Could you check a few things on this model? Use its own coordinates, in mm. Face numbers are marked on the shaded views. Round coordinates to 2 decimals unless told otherwise and drop trailing zeros. Loops run counter-clockwise (first coordinate to the right, second up) from the corner with the lowest first, then second, coordinate; pieces in that order, holes last. Notation, with made-up numbers: M -22.75,17.5 L 9.25,17.5 A19 ccw 9.25,38.5 Z; hole C 85.5,-27.75 d11. An arc over 180 degrees is marked long. One line per item, written item: value. Start each with the question number.
Q1. Imagine slicing it at B-B (z = 4.5). Please give me the cut outline in (x, y).
Q2. Imagine slicing it at D-D (z = 9.25). Give the number of separate pieces and of enclosed holes in the cut face, then the cut area to 3 significant figures.
Q3. Imagine slicing it at A-A (y = 51). Please give me the cut outline in (x, z), then the cut area to 3 significant figures.
Q4. Imagine slicing it at C-C (x = 21). Please give me the cut outline in (y, z), then the cut area to 3 significant figures.
Q5. I'm going to push flat-ended pins straight in: pin 1 Ø2 at (x, y) = (20.5, 37) entering from +Z; pin 2 Ø5 at (x, z) = (5.5, 6) entering from +Y; pin 3 Ø1 at (x, z) = (6.5, 3) entering from -Y. Where does each tip first touch, or does it pass through?
Q6. Please list where these lines run through material, in increasing order: line 1 along X through (y, z) = (39, 8.5); line 2 along X through (y, z) = (20, 8.25); line 3 along Y through (x, z) = (22, 8.25).
Q7. Thinking about a two-plate mould opening in X: for the marked faces 1, 2, 3 and 4, which applies, released by +X, released by -X, zero draft, split by the parting line, or undercut?
from build123d import *

# Parameters (mm, degrees)
EXTRUDE1_DEPTH = 10.16
CHAMFER1_SIZE  = 2.54
FILLET1_R      = 2.54
SKETCH2_R      = 2.50622178
SKETCH2_W      = 20.082955398
SKETCH2_H      = 27.0305724
EXTRUDE2_DEPTH = 2.54
FILLET2_R      = 5.08


with BuildPart() as part:
    # Sketch1 → Extrude1 (new body)
    with BuildSketch(Plane.XY):
        with BuildLine():
            Line((10.16, 0), (30.130017372, 0))
            ThreePointArc((30.130017372, 0), (37.314222268, 2.975795103), (40.290017372, 10.16))
            Line((40.290017372, 10.16), (40.290017372, 70.869919512))
            ThreePointArc((40.290017372, 70.869919512), (37.314222268, 78.054124409), (30.130017372, 81.029919512))
            Line((30.130017372, 81.029919512), (10.16, 81.029919512))
            ThreePointArc((10.16, 81.029919512), (2.975795103, 78.054124409), (0, 70.869919512))
            Line((0, 70.869919512), (0, 10.16))
            ThreePointArc((0, 10.16), (2.975795103, 2.975795103), (10.16, 0))
        make_face()
    extrude(amount=EXTRUDE1_DEPTH)

    # Chamfer1
    chamfer1_edges = [part.edges().sort_by_distance(p)[0] for p in [
        (2.975795103, 2.975795103, 10.16),
        (20.145008686, 0, 10.16),
        (37.314222268, 2.975795103, 10.16),
        (40.290017372, 40.514959756, 10.16),
        (37.314222268, 78.054124409, 10.16),
        (20.145008686, 81.029919512, 10.16),
        (2.975795103, 78.054124409, 10.16),
        (0, 40.514959756, 10.16),
    ]]
    chamfer(chamfer1_edges, length=CHAMFER1_SIZE)

    # Fillet1
    fillet1_edges = [part.edges().sort_by_distance(p)[0] for p in [
        (0, 40.514959756, 0),
        (2.975795103, 78.054124409, 0),
        (20.145008686, 81.029919512, 0),
        (37.314222268, 78.054124409, 0),
        (40.290017372, 40.514959756, 0),
        (37.314222268, 2.975795103, 0),
        (20.145008686, 0, 0),
        (2.975795103, 2.975795103, 0),
    ]]
    fillet(fillet1_edges, radius=FILLET1_R)

    # Sketch2 → Extrude2 (cut)
    with BuildSketch(Plane.XY.offset(10.16)):
        with Locations((10.754870081, 36.715481708)):
            Circle(SKETCH2_R)
        with Locations((20.03645217, 36.715481708)):
            Circle(SKETCH2_R)
        with Locations((29.318034259, 36.715481708)):
            Circle(SKETCH2_R)
        with Locations((10.754870081, 29.095481708)):
            Circle(SKETCH2_R)
        with Locations((20.03645217, 29.095481708)):
            Circle(SKETCH2_R)
        with Locations((29.318034259, 29.095481708)):
            Circle(SKETCH2_R)
        with Locations((10.754870081, 21.475481708)):
            Circle(SKETCH2_R)
        with Locations((20.03645217, 21.475481708)):
            Circle(SKETCH2_R)
        with Locations((29.318034259, 21.475481708)):
            Circle(SKETCH2_R)
        with Locations((10.754870081, 13.855481708)):
            Circle(SKETCH2_R)
        with Locations((20.03645217, 13.855481708)):
            Circle(SKETCH2_R)
        with Locations((29.318034259, 13.855481708)):
            Circle(SKETCH2_R)
        with Locations((20.03645217, 57.286941426)):
            Rectangle(SKETCH2_W, SKETCH2_H)
    extrude(amount=-EXTRUDE2_DEPTH, mode=Mode.SUBTRACT)

    # Fillet2
    fillet2_edges = [part.edges().sort_by_distance(p)[0] for p in [
        (9.994974471, 43.771655226, 8.89),
        (9.994974471, 70.802227626, 8.89),
        (30.077929869, 70.802227626, 8.89),
        (30.077929869, 43.771655226, 8.89),
    ]]
    fillet(fillet2_edges, radius=FILLET2_R)


solid = part.part
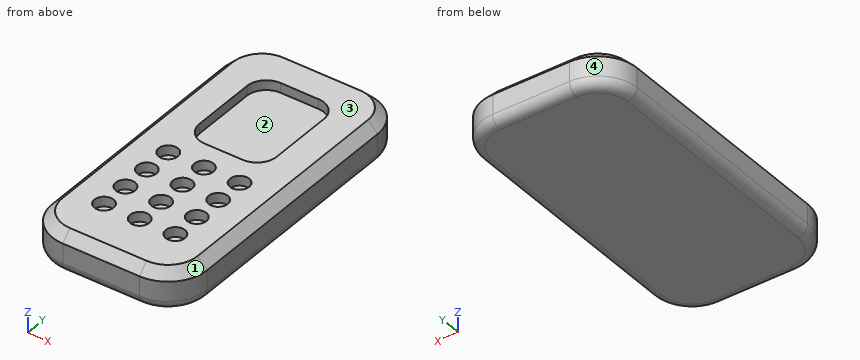
Report:
1. outline: M 0,10.16 A10.16 ccw 10.16,0 L 30.13,0 A10.16 ccw 40.29,10.16 L 40.29,70.87 A10.16 ccw 30.13,81.03 L 10.16,81.03 A10.16 ccw 0,70.87 Z
2. separate pieces: 1
2. enclosed holes: 13
2. area: 2,060 mm²
3. outline: M 0,2.54 A2.54 ccw 2.54,0 L 37.75,0 A2.54 ccw 40.29,2.54 L 40.29,7.62 L 37.75,10.16 L 30.08,10.16 L 30.08,7.62 L 9.99,7.62 L 9.99,10.16 L 2.54,10.16 L 0,7.62 Z
3. area: 349 mm²
4. outline: M 0,2.54 A2.54 ccw 2.54,0 L 78.49,0 A2.54 ccw 81.03,2.54 L 81.03,7.62 L 78.49,10.16 L 70.8,10.16 L 70.8,7.62 L 43.77,7.62 L 43.77,10.16 L 39.03,10.16 L 39.03,7.62 L 34.4,7.62 L 34.4,10.16 L 31.41,10.16 L 31.41,7.62 L 26.78,7.62 L 26.78,10.16 L 23.79,10.16 L 23.79,7.62 L 19.16,7.62 L 19.16,10.16 L 16.17,10.16 L 16.17,7.62 L 11.54,7.62 L 11.54,10.16 L 2.54,10.16 L 0,7.62 Z
4. area: 698 mm²
5. pin 1: stops at z = 7.62
5. pin 2: stops at y = 80.8
5. pin 3: stops at y = 0.5
6. line 1: x = 0.88 to 9.72, 11.79 to 19.01, 21.07 to 28.29, 30.35 to 39.41
6. line 2: x = 0.63 to 8.73, 12.78 to 18.01, 22.06 to 27.29, 31.34 to 39.66
6. line 3: y = 0.63 to 12.3, 15.41 to 19.92, 23.03 to 27.54, 30.65 to 35.16, 38.27 to 43.77, 70.8 to 80.4
7. face 1: released by +X
7. face 2: undercut
7. face 3: zero draft
7. face 4: released by -X
